Study the drawing (mm; zero at the part's minimum x, y, z) and answer. Give positions to 0.01 mm unless a question says otherwise; leave off trailing zeros. Order: outer loops, then holes, each group sorted by start corner. A loop starts at its lowest first (then second) coordinate and runs counter-clockwise, first axis right, second up. Notation, with made-up numbers: (-12.75, 7) -> (2.25, 7) arc R20 cw to (2.25, 26) -> close; hole circle Ø3 at (78.5, 8.25). An arc over 180 degrees is marked (long way). One line per question, with ' | ' between items. Start each with the question number.
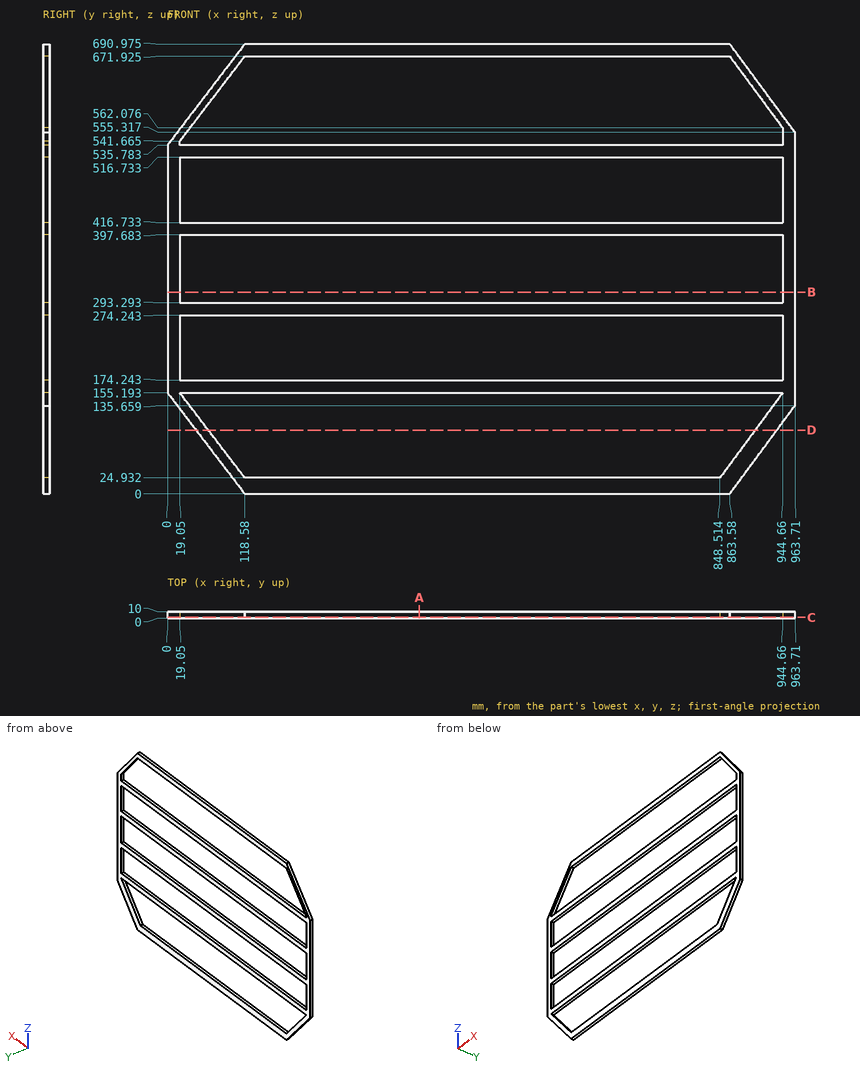
Q1. A cutting plane is placed at A-A, the plane x = 387. Determine the outline of the cut face in (y, z) (1 decimal).
Q2. Find the intervals of material crossed by line 1 (Z direction, x = 307.5, y = 4.25) (1 decimal); line 2 (X direction, y = 6, z = 217.5); line 3 (Z direction, x = 62.5, y = 2.5) (1 decimal), in increasing order.
Q3. A cutting plane is placed at C-C, the plane y = 1.75. Give the number of separate pieces and of enclosed holes in the cut face, then the cut area to 3 significant figures.
Q4. A cutting plane is placed at B-B, the plane z = 310. Determine the outline of the cut face in (x, y), then the cut area to 3 significant figures.
Q5. Given P1, Ø1, axis at y = 6, z = 78.5, coming from the -X side, flat-ended and moving along its own axis, determine where the tip first touches the part or whether it passes through.
Q6. A cutting plane is placed at D-D, the plane z = 98. Determine the outline of the cut face in (x, y), then the cut area to 3 significant figures.
Geometry results:
1) outline: (0, 0) -> (10, 0) -> (10, 24.9) -> (0, 24.9) -> close; (0, 155.2) -> (10, 155.2) -> (10, 174.2) -> (0, 174.2) -> close; (0, 274.2) -> (10, 274.2) -> (10, 293.3) -> (0, 293.3) -> close; (0, 397.7) -> (10, 397.7) -> (10, 416.7) -> (0, 416.7) -> close; (0, 516.7) -> (10, 516.7) -> (10, 535.8) -> (0, 535.8) -> close; (0, 671.9) -> (10, 671.9) -> (10, 691) -> (0, 691) -> close
2) line 1: 0 to 24.9, 155.2 to 174.2, 274.2 to 293.3, 397.7 to 416.7, 516.7 to 535.8, 671.9 to 691 | line 2: 0 to 19.05, 944.66 to 963.71 | line 3: 73.4 to 98.3, 155.2 to 174.2, 274.2 to 293.3, 397.7 to 416.7, 516.7 to 535.8, 598.5 to 617.6
3) separate pieces: 1 | enclosed holes: 5 | area: 129,000 mm²
4) outline: (0, 0) -> (19.05, 0) -> (19.05, 10) -> (0, 10) -> close; (944.66, 0) -> (963.71, 0) -> (963.71, 10) -> (944.66, 10) -> close | area: 381 mm²
5) P1: x = 58.22
6) outline: (43.7, 0) -> (62.75, 0) -> (62.75, 10) -> (43.7, 10) -> close; (902.45, 0) -> (935.91, 0) -> (935.91, 10) -> (902.45, 10) -> close | area: 525 mm²
